Design review of the part shown in the three views and the two pictorial views. Dimensions are in mm from the part's minimum x, y and z. A direction names the side the tool comes from. Round coordinates to 2 decimals unless told otherwise and drop trailing zeros. Order: outer loops, then holes, each group sorted by start corner. A loop starts at its lowest first (then second) coordinate and runs counter-clockwise, first axis right, second up.
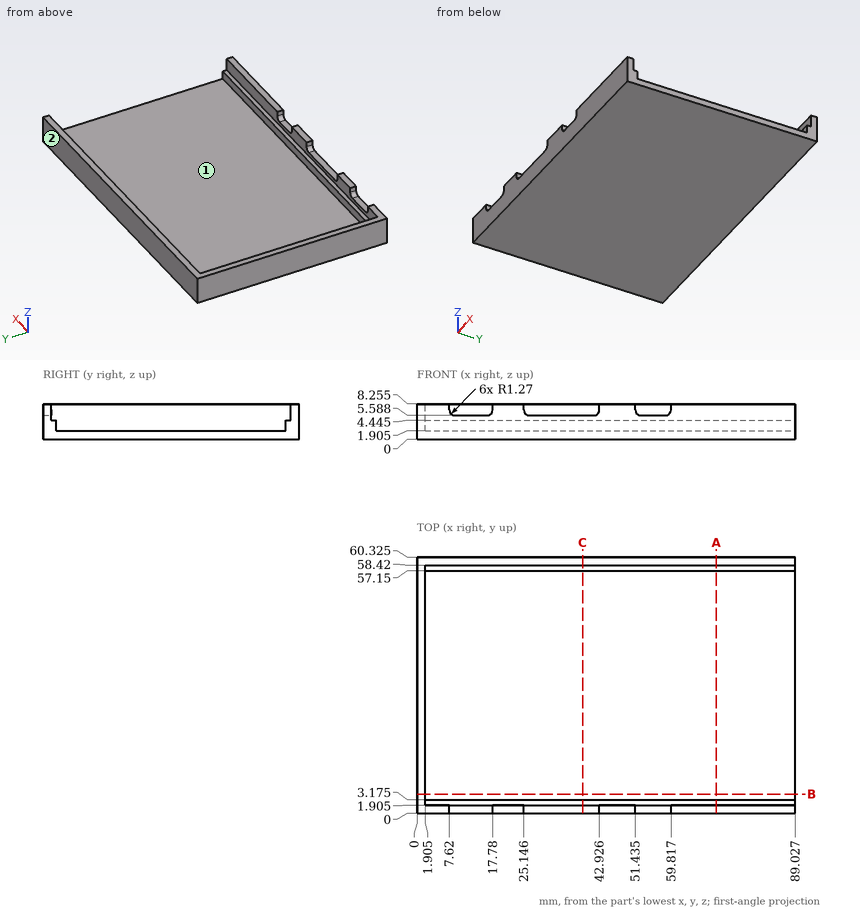
(1) Add section B-B on y = 4.5. Give the boundary of the cut face in (x, z) (3 decimals), plus the area to 3 significant figures.
(2) Wall thickness on L1, parallel to Y at x = 8, z = 3.5 (3 decimals); L2, parallel to Y at x = 69, z = 7 (3 decimals); L3, parallel to Z at x = 47.5, y = 18 (3 decimals): over which ranges is each line inside the solid? List them lowest first.
(3) Clearance check with flat-ended pins moving along their axes: P1, Ø4, axis at x = 26.5, y = 51.5, coming from the -Z side; P2, Ø1, axis at x = 29.5, y = 2.5, coming from the +Z side (3 decimals); P3, Ø1, axis at x = 56.5, y = 1, coming from the +Z side; P4, Ø12, axis at x = 39.5, y = 32.5, coming from the +Z side (3 decimals). State where each tip first meets the part, or that it passes through.
(4) Add section C-C on x = 39. Give the boundary of the cut face in (y, z) (3 decimals), plus the area to 3 significant figures.
(5) Add section A-A on x = 70.5. Give the boundary of the cut face in (y, z) (3 decimals).
(6) Tool access review of the marked faces 1 and 2: name each direction out of +Z, -Z, +X, -X, +Y, -Y from which nothing blocks a thin tool from reaching the whole face with its end or side.
Here are the results:
1. outline: (0, 0) - (89.027, 0) - (89.027, 1.905) - (1.905, 1.905) - (1.905, 8.255) - (0, 8.255) - close
1. area: 182 mm2
2. L1: y = 0 to 3.175, 57.15 to 60.325
2. L2: y = 0 to 1.905, 58.42 to 60.325
2. L3: z = 0 to 1.905
3. P1: stops at z = 0
3. P2: stops at z = 4.445
3. P3: stops at z = 5.59
3. P4: stops at z = 1.905
4. outline: (0, 0) - (60.325, 0) - (60.325, 8.255) - (58.42, 8.255) - (58.42, 4.445) - (57.15, 4.445) - (57.15, 1.905) - (3.175, 1.905) - (3.175, 4.445) - (1.905, 4.445) - (1.905, 5.588) - (0, 5.588) - close
4. area: 140 mm2
5. outline: (0, 0) - (60.325, 0) - (60.325, 8.255) - (58.42, 8.255) - (58.42, 4.445) - (57.15, 4.445) - (57.15, 1.905) - (3.175, 1.905) - (3.175, 4.445) - (1.905, 4.445) - (1.905, 8.255) - (0, 8.255) - close
6. face 1: +Z, +X
6. face 2: +Z, -Z, +X, -X, +Y
